Build history of the part. All positions in model axes, mm. Face numbers are marked on the shaded views. Coordinates: 2 decimals unless noted, no trailing zeros. Write each loop counter-clockwise with the first axis right and the second up, starting at its lowest first coordinate (ties: lowest second). Pieces come first, ordered by that corner, then holes.
from build123d import *

# Parameters (mm, degrees)
SKETCH1_R           = 16
SKETCH1_R_2         = 14
BOSS_EXTRUDE1_DEPTH = 30
BOSS_EXTRUDE3_START = -2
SKETCH3_R           = 14
SKETCH3_R_2         = 12
BOSS_EXTRUDE3_DEPTH = 2
CHAMFER1_SIZE       = 2
BOSS_EXTRUDE4_START = 2
SKETCH4_R           = 19
SKETCH4_R_2         = 16
BOSS_EXTRUDE4_DEPTH = 2
FILLET2_R           = 10


# Some blends are built 0.0001 mm under size
with BuildPart() as part:
    # Sketch1 → Boss-Extrude1 (new body)
    with BuildSketch(Plane(origin=(0, 0, 0), x_dir=(1, 0, 0), z_dir=(0, 1, 0))):
        with Locations(Location((0, 0, 0), (0, 0, 270))):
            Circle(SKETCH1_R)
        with Locations(Location((0, 0, 0), (0, 0, 270))):
            Circle(SKETCH1_R_2, mode=Mode.SUBTRACT)
    extrude(amount=BOSS_EXTRUDE1_DEPTH)

    # Sketch3 → Boss-Extrude3 (add)
    with BuildSketch(Plane(origin=(0, 27, 0), x_dir=(1, 0, 0), z_dir=(0, 1, 0)).offset(BOSS_EXTRUDE3_START)):
        with Locations(Location((0, 0, 0), (0, 0, 270))):
            Circle(SKETCH3_R)
        with Locations(Location((0, 0, 0), (0, 0, 270))):
            Circle(SKETCH3_R_2, mode=Mode.SUBTRACT)
    extrude(amount=BOSS_EXTRUDE3_DEPTH)

    # Chamfer1
    chamfer1_edges = [part.edges().sort_by_distance(p)[0] for p in [
        (0, 25, -14),
    ]]
    chamfer(chamfer1_edges, length=CHAMFER1_SIZE - 0.0001)  # a hair under: the kernel refuses the full size

    # Sketch4 → Boss-Extrude4 (add)
    with BuildSketch(Plane(origin=(0, 2, 0), x_dir=(-1, 0, 0), z_dir=(0, -1, 0)).offset(BOSS_EXTRUDE4_START)):
        with Locations(Location((0, 0, 0), (0, 0, 270))):
            Circle(SKETCH4_R)
        with Locations(Location((0, 0, 0), (0, 0, 90))):
            Circle(SKETCH4_R_2, mode=Mode.SUBTRACT)
    extrude(amount=-BOSS_EXTRUDE4_DEPTH)

    # Fillet2
    # the kernel refuses this fillet: 10 mm, written as the material it adds along each edge
    with BuildSketch(Plane(origin=(0, 2, 0), x_dir=(0, 0, 1), z_dir=(1, 0, 0))) as fillet2_piece_1:
        with BuildLine():
            CenterArc((26, -7.141428429), FILLET2_R, 134.427004001, 45.572995999)
            Line((16, -7.141428429), (15.8, -7.141428429))
            Line((15.8, -7.141428429), (15.8, 0))
            Line((15.8, 0), (16, 0.2))
            ThreePointArc((16, 0.2), (17.5, 0.2), (18.86, 0.142828569))
            Line((18.86, 0.142828569), (19, 0))
        make_face()
    revolve(axis=Axis((0, 2, 0), (0, -1, 0)))


solid = part.part
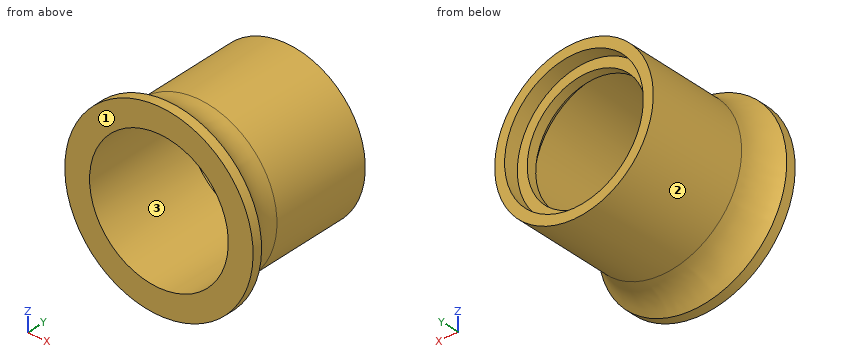
(1) Slice it at C-C, the plane y = 11. List the corners of the cut face in (x, z), and give its area (3 significant figures).
(2) Slice it at D-D, the plane y = 4.75. List the corners of the cut face in (x, z).
(3) Two-plate mould, pull along X, no slides. Class the marked faces 1, 2 and 3: pulls with the +X half, pulls with the -X half, needs draft (parallel to the pull), parting line crosses it, or undercut.
(4) Flat gauge pins, fed straight in: P1, Ø10, axis at y = 16.5, z = 12, coming from the +X side; P2, Ø10, axis at y = 6.5, z = -5.5, coming from the -X side; P3, Ø10, axis at x = 8.5, y = 7, coming from the +Z side. Where does each tip first touch, or does it go through?
(5) Probe L1, parallel to X at y = 29.2, z = 0; L2, parallel to Z at x = -8.5, y = 4; L3, parallel to X at y = 18.75, z = 8.5. List the from-to ranges inside material, lowest first.
Results:
1. outline: circle Ø32 at (0, 0); hole circle Ø28 at (0, 0)
1. area: 188 mm2
2. outline: circle Ø34.03 at (0, 0); hole circle Ø28 at (0, 0)
3. face 1: needs draft
3. face 2: parting line crosses it
3. face 3: undercut
4. P1: stops at x = 14.39
4. P2: stops at x = -18.71
4. P3: stops at z = 17.43
5. L1: x = -16 to -14, 14 to 16
5. L2: z = -15.21 to -11.12, 11.12 to 15.21
5. L3: x = -13.56 to -11.12, 11.12 to 13.56
